```python
from build123d import *

# Parameters (mm, degrees)
F0_W      = 40
F0_H      = 500
F1_DEPTH  = 3
F3_D      = 8
F5_D      = 12
F7_DEPTH  = 6
F8_D      = 12
F10_DEPTH = 6
F12_DEPTH = 6
F13_R     = 5
F15_D     = 6


with BuildPart() as f1:
    # F0 (on Front) → F1 (new body)
    with BuildSketch(Plane.XZ):
        Rectangle(F0_W, F0_H)
    extrude(amount=F1_DEPTH)

    # F3 (through all)
    with Locations(Plane.XZ.offset(3)):
        with Locations((0, -215), (0, 215)):
            Hole(F3_D / 2)

    # F5 (through all)
    with Locations(Plane.XZ.offset(3)):
        with Locations((0, 149)):
            Hole(F5_D / 2)

    # F6 (on face) → F7 (cut)
    with BuildSketch(Plane.XZ.offset(3)):
        with BuildLine():
            ThreePointArc((-3, 155), (0, 152), (3, 155))
            Line((3, 155), (3, 175))
            ThreePointArc((3, 175), (0, 178), (-3, 175))
            Line((-3, 175), (-3, 155))
        make_face()
    extrude(amount=-F7_DEPTH, mode=Mode.SUBTRACT)

    # F8 (through all)
    with Locations(Plane.XZ.offset(3)):
        with Locations((0, -178.25)):
            Hole(F8_D / 2)

    # F9 (on face) → F10 (cut)
    with BuildSketch(Plane.XZ.offset(3)):
        with BuildLine():
            ThreePointArc((-3, -172.25), (0, -175.25), (3, -172.25))
            Line((3, -172.25), (3, -152.25))
            ThreePointArc((3, -152.25), (0, -149.25), (-3, -152.25))
            Line((-3, -152.25), (-3, -172.25))
        make_face()
    extrude(amount=-F10_DEPTH, mode=Mode.SUBTRACT)

    # F11 (on face) → F12 (cut)
    with BuildSketch(Plane.XZ.offset(3)):
        with BuildLine():
            ThreePointArc((-6, 149), (0, 143), (6, 149))
            Line((6, 149), (6, 175))
            ThreePointArc((6, 175), (0, 181), (-6, 175))
            Line((-6, 175), (-6, 149))
        make_face()
        with BuildLine():
            ThreePointArc((-6, -178.25), (0, -184.25), (6, -178.25))
            Line((6, -178.25), (6, -152.25))
            ThreePointArc((6, -152.25), (0, -146.25), (-6, -152.25))
            Line((-6, -152.25), (-6, -178.25))
        make_face()
    extrude(amount=-F12_DEPTH, mode=Mode.SUBTRACT)

    # F13
    f13_edges = [f1.edges().sort_by_distance(p)[0] for p in [
        (20, -1.5, 250),
        (-20, -1.5, 250),
        (20, -1.5, -250),
        (-20, -1.5, -250),
    ]]
    fillet(f13_edges, radius=F13_R)

    # F15 (through all)
    with Locations(Plane.XZ.offset(3)):
        with Locations((0, 20), (0, -20)):
            Hole(F15_D / 2)


solid = f1.part
```
Source: CAD feature listing. Evaluate the final solid. Frame: model axes, mm. Give positions to 0.01 mm unless a question says otherwise; leave off trailing zeros. Order: outer loops, then holes, each group sorted by start corner. A loop starts at its lowest first (then second) coordinate and runs counter-clockwise, first axis right, second up.
(1) Pull-direction query (X, two-part tool) for faces 1 (the face through (0, 0, 4)), 2 (the face through (0.521, -1.479, -211.034)); classes: +X half, -X half, draft (parallel to the pull), parting line (faces both ways), or undercut.
(2) Contact query for a flat-ended pin moving along its axis: P1, Ø5, axis at x = 0, z = 20, coming from the +Y side. Output: stop coordinate, or through.
(3) Section query B-B (z = 154). Return the cut outline in (x, y), plus the area to 3 significant figures.
(4) Section query A-A (y = -1.65). Return the cut outline in (x, z).
(5) Material intervals for line 1 along X through (y, z) = (-0.75, 150); line 2 along X through (y, z) = (-0.9, -181); line 3 along Z through (x, y) = (-18, -2.8), sorted ascending.
Outcome:
1. face 1: draft
1. face 2: undercut
2. P1: passes through
3. outline: (-20, -3) - (-6, -3) - (-6, 0) - (-20, 0) - close; (6, -3) - (20, -3) - (20, 0) - (6, 0) - close
3. area: 84.0 mm2
4. outline: (-20, -245) arc R5 ccw to (-15, -250) - (15, -250) arc R5 ccw to (20, -245) - (20, 245) arc R5 ccw to (15, 250) - (-15, 250) arc R5 ccw to (-20, 245) - close; hole (-6, -178.25) arc R6 ccw to (6, -178.25) - (6, -152.25) arc R6 ccw to (-6, -152.25) - close; hole (-6, 149) arc R6 ccw to (6, 149) - (6, 175) arc R6 ccw to (-6, 175) - close; hole circle Ø8 at (0, -215); hole circle Ø8 at (0, 215); hole circle Ø6 at (0, -20); hole circle Ø6 at (0, 20)
5. line 1: x = -20 to -6, 6 to 20
5. line 2: x = -20 to -5.33, 5.33 to 20
5. line 3: z = -249 to 249
